The listing builds one solid part. Answer for the finished solid, in the listing's coordinates (mm). Round coordinates to 2 decimals unless told otherwise and drop trailing zeros. Write each loop counter-clockwise with the first axis right and the second up, starting at its lowest first coordinate (ties: lowest second). Pieces come first, ordered by that corner, then holes. Notation, with made-up numbers: (26, 67) - (70, 67) arc R6 ccw to (70, 76) - close; hole circle Ø3 at (-24, 52). An arc over 180 degrees is marked (long way). Answer as CSV lines item,"result". Start each with the question number.
Item 1: Flat-ended cylindrical pins translate along their axes: pin 1 (1 mm diameter, centred on x = -13.5, z = 39, fed in from -Y); pin 2 (2 mm diameter, centred on x = 33, y = 13.5, fed in from +Z); pin 3 (2 mm diameter, centred on x = 11.5, y = -21.5, fed in from -Z). Find the tip coordinate at first contact, or state that the pin passes through.
Item 2: A cutting plane is placed at A-A on y = 7. Determine the outline of the cut face in (x, z), and give its area (3 significant figures).
Item 3: Straight lines are drawn through the part: line 1 along Z through (x, y) = (28.5, 29); line 2 along Z through (x, y) = (30.5, -8); line 3 along Y through (x, z) = (-17, 26.5). For each, find the intervals that lie inside material, in ascending order. Write a range as [from, to].
Item 4: A cutting plane is placed at B-B on z = -24. Determine the outline of the cut face in (x, y).
Item 5: A cutting plane is placed at C-C on x = 32. Determine the outline of the cut face in (y, z).
Item 6: A cutting plane is placed at D-D on y = 31.5. Determine the outline of the cut face in (x, z), and give its area (3 significant figures).
```python
from build123d import *

# Parameters (mm, degrees)
F12_DEPTH      = 37.3243635206
F12_DEPTH_BACK = 37.3243635206
F15_DEPTH      = 37.3243635206
F15_DEPTH_BACK = 37.3243635206
F18_DEPTH      = 37.3243635206
F18_DEPTH_BACK = 37.3243635206
F21_DEPTH      = 37.3243635206
F21_DEPTH_BACK = 37.3243635206
F24_DEPTH      = 37.3243635206
F24_DEPTH_BACK = 37.3243635206
F28_DEPTH      = 99.1671965959
F28_DEPTH_BACK = 99.1671965959
F32_DEPTH      = 89.4601183415
F32_DEPTH_BACK = 89.4601183415
F35_DEPTH      = 89.4601183415
F35_DEPTH_BACK = 88.5596960493
F39_DEPTH      = 99.1671965959
F39_DEPTH_BACK = 96.8098604305
F42_DEPTH      = 68.0823305395
F42_DEPTH_BACK = 70.9961582856
F45_DEPTH      = 92.4043169267
F45_DEPTH_BACK = 99.1671965959
F48_DEPTH      = 81.4313769211
F48_DEPTH_BACK = 89.4601183415
F52_DEPTH      = 88.5596960493
F52_DEPTH_BACK = 82.3317992133
F56_DEPTH      = 92.4043169267
F56_DEPTH_BACK = 96.8098604305
F59_DEPTH      = 68.0823305395
F59_DEPTH_BACK = 68.0823305395
F62_DEPTH      = 37.3243635206
F62_DEPTH_BACK = 37.3243635206
F65_DEPTH      = 68.0823305395
F65_DEPTH_BACK = 68.0823305395
F68_DEPTH      = 81.4313769211
F68_DEPTH_BACK = 81.4313769211
F71_DEPTH      = 92.4043169267
F71_DEPTH_BACK = 92.4043169267
F74_DEPTH      = 92.4043169267
F74_DEPTH_BACK = 92.4043169267


# Not quite as in the source:
# - a feature names something its author has since deleted; it is built from what else it names


with BuildPart() as f9:
    # F7 (on Front) → F9 (revolve)
    with BuildSketch(Plane.XZ):
        with BuildLine():
            Line((0, 0), (0, 31.75))
            Line((0, 31.75), (0, 70.9951582856))
            ThreePointArc((0, 70.9951582856), (-70.9951582856, 0), (0, -70.9951582856))
            Line((0, -70.9951582856), (0, -31.75))
            Line((0, -31.75), (0, 0))
        make_face()
    revolve(axis=Axis((0, 0, -35.4975791428), (0, 0, -1)))

    # F11 (on 3pt) → F12 (cut, two sides)
    with BuildSketch(Plane(origin=(0, 0, 0), x_dir=(-0.5877852523, 0.8090169944, 0), z_dir=(0.8090169944, 0.5877852523, 0))) as f12_sk:
        Polygon((-63.5, -70.9951582856), (0, -70.9951582856), (-51.3725791428, -31.75), (-63.5, -31.75), align=None)
    extrude(amount=F12_DEPTH, mode=Mode.SUBTRACT)
    extrude(f12_sk.sketch, amount=-F12_DEPTH_BACK, mode=Mode.SUBTRACT)

    # F14 (on 3pt) → F15 (cut, two sides)
    with BuildSketch(Plane(origin=(0, 0, 0), x_dir=(-0.5877852523, -0.8090169944, 0), z_dir=(-0.8090169944, 0.5877852523, 0))) as f15_sk:
        Polygon((51.3725791428, -31.75), (0, -70.9951582856), (63.5, -70.9951582856), (63.5, -31.75), align=None)
    extrude(amount=-F15_DEPTH, mode=Mode.SUBTRACT)
    extrude(f15_sk.sketch, amount=F15_DEPTH_BACK, mode=Mode.SUBTRACT)

    # F17 (on 3pt) → F18 (cut, two sides)
    with BuildSketch(Plane(origin=(0, 0, 0), x_dir=(0.9510565163, -0.3090169944, 0), z_dir=(-0.3090169944, -0.9510565163, 0))) as f18_sk:
        Polygon((-63.5, -70.9951582856), (0, -70.9951582856), (-51.3725791428, -31.75), (-63.5, -31.75), align=None)
    extrude(amount=-F18_DEPTH, mode=Mode.SUBTRACT)
    extrude(f18_sk.sketch, amount=F18_DEPTH_BACK, mode=Mode.SUBTRACT)

    # F20 (on 3pt) → F21 (cut, two sides)
    with BuildSketch(Plane.YZ) as f21_sk:
        Polygon((51.3725791428, -31.75), (0, -70.9951582856), (63.5, -70.9951582856), (63.5, -31.75), align=None)
    extrude(amount=-F21_DEPTH, mode=Mode.SUBTRACT)
    extrude(f21_sk.sketch, amount=F21_DEPTH_BACK, mode=Mode.SUBTRACT)

    # F23 (on 3pt) → F24 (cut, two sides)
    with BuildSketch(Plane(origin=(0, 0, 0), x_dir=(-0.9510565163, -0.3090169944, 0), z_dir=(-0.3090169944, 0.9510565163, 0))) as f24_sk:
        Polygon((-63.5, -70.9951582856), (0, -70.9951582856), (-51.3725791428, -31.75), (-63.5, -31.75), align=None)
    extrude(amount=F24_DEPTH, mode=Mode.SUBTRACT)
    extrude(f24_sk.sketch, amount=-F24_DEPTH_BACK, mode=Mode.SUBTRACT)

    # F27 (on 3pt) → F28 (cut, two sides)
    with BuildSketch(Plane(origin=(0, 0, 0), x_dir=(-0.5877852523, 0.8090169944, 0), z_dir=(0.8090169944, 0.5877852523, 0))) as f28_sk:
        Polygon((-70.9951582856, -31.75), (-51.3725791428, -31.75), (-63.5, 31.75), (-70.9951582856, 31.75), align=None)
    extrude(amount=F28_DEPTH, mode=Mode.SUBTRACT)
    extrude(f28_sk.sketch, amount=-F28_DEPTH_BACK, mode=Mode.SUBTRACT)

    # F31 (on 3pt) → F32 (cut, two sides)
    with BuildSketch(Plane(origin=(0, 0, 0), x_dir=(0.9510565163, -0.3090169944, 0), z_dir=(-0.3090169944, -0.9510565163, 0))) as f32_sk:
        Polygon((70.9951582856, 31.75), (51.3725791428, 31.75), (63.5, -31.75), (70.9951582856, -31.75), align=None)
    extrude(amount=-F32_DEPTH, mode=Mode.SUBTRACT)
    extrude(f32_sk.sketch, amount=F32_DEPTH_BACK, mode=Mode.SUBTRACT)

    # F34 (on 3pt) → F35 (cut, two sides)
    with BuildSketch(Plane(origin=(0, 0, 0), x_dir=(0.9510565163, 0.3090169944, 0), z_dir=(0.3090169944, -0.9510565163, 0))) as f35_sk:
        Polygon((63.5, 31.75), (51.3725791428, -31.75), (70.9951582856, -31.75), (70.9951582856, 31.75), align=None)
    extrude(amount=-F35_DEPTH, mode=Mode.SUBTRACT)
    extrude(f35_sk.sketch, amount=F35_DEPTH_BACK, mode=Mode.SUBTRACT)

    # F38 (on 3pt) → F39 (cut, two sides)
    with BuildSketch(Plane(origin=(0, 0, 0), x_dir=(0.5877852523, 0.8090169944, 0), z_dir=(0.8090169944, -0.5877852523, 0))) as f39_sk:
        Polygon((70.9951582856, 31.75), (51.3725791428, 31.75), (63.5, -31.75), (70.9951582856, -31.75), align=None)
    extrude(amount=-F39_DEPTH, mode=Mode.SUBTRACT)
    extrude(f39_sk.sketch, amount=F39_DEPTH_BACK, mode=Mode.SUBTRACT)

    # F41 (on 3pt) → F42 (cut, two sides)
    with BuildSketch(Plane(origin=(0, 0, 0), x_dir=(0, -1, 0), z_dir=(-1, 0, 0))) as f42_sk:
        Polygon((-70.9951582856, -31.75), (-51.3725791428, -31.75), (-63.5, 31.75), (-70.9951582856, 31.75), align=None)
    extrude(amount=-F42_DEPTH, mode=Mode.SUBTRACT)
    extrude(f42_sk.sketch, amount=F42_DEPTH_BACK, mode=Mode.SUBTRACT)

    # F44 (on 3pt) → F45 (cut, two sides)
    with BuildSketch(Plane(origin=(0, 0, 0), x_dir=(0.5877852523, -0.8090169944, 0), z_dir=(-0.8090169944, -0.5877852523, 0))) as f45_sk:
        Polygon((-63.5, -31.75), (-51.3725791428, 31.75), (-70.9951582856, 31.75), (-70.9951582856, -31.75), align=None)
    extrude(amount=-F45_DEPTH, mode=Mode.SUBTRACT)
    extrude(f45_sk.sketch, amount=F45_DEPTH_BACK, mode=Mode.SUBTRACT)

    # F47 (on 3pt) → F48 (cut, two sides)
    with BuildSketch(Plane(origin=(0, 0, 0), x_dir=(0.9510565163, -0.3090169944, 0), z_dir=(-0.3090169944, -0.9510565163, 0))) as f48_sk:
        Polygon((-70.9951582856, -31.75), (-51.3725791428, -31.75), (-63.5, 31.75), (-70.9951582856, 31.75), align=None)
    extrude(amount=-F48_DEPTH, mode=Mode.SUBTRACT)
    extrude(f48_sk.sketch, amount=F48_DEPTH_BACK, mode=Mode.SUBTRACT)

    # F51 (on 3pt) → F52 (cut, two sides)
    with BuildSketch(Plane(origin=(0, 0, 0), x_dir=(-0.9510565163, -0.3090169944, 0), z_dir=(-0.3090169944, 0.9510565163, 0))) as f52_sk:
        Polygon((70.9951582856, 31.75), (51.3725791428, 31.75), (63.5, -31.75), (70.9951582856, -31.75), align=None)
    extrude(amount=-F52_DEPTH, mode=Mode.SUBTRACT)
    extrude(f52_sk.sketch, amount=F52_DEPTH_BACK, mode=Mode.SUBTRACT)

    # F55 (on 3pt) → F56 (cut, two sides)
    with BuildSketch(Plane(origin=(0, 0, 0), x_dir=(0.5877852523, 0.8090169944, 0), z_dir=(0.8090169944, -0.5877852523, 0))) as f56_sk:
        Polygon((-70.9951582856, -31.75), (-51.3725791428, -31.75), (-63.5, 31.75), (-70.9951582856, 31.75), align=None)
    extrude(amount=-F56_DEPTH, mode=Mode.SUBTRACT)
    extrude(f56_sk.sketch, amount=F56_DEPTH_BACK, mode=Mode.SUBTRACT)

    # F58 (on 3pt) → F59 (cut, two sides)
    with BuildSketch(Plane(origin=(0, 0, 0), x_dir=(0, -1, 0), z_dir=(-1, 0, 0))) as f59_sk:
        Polygon((70.9951582856, 31.75), (51.3725791428, 31.75), (63.5, -31.75), (70.9951582856, -31.75), align=None)
    extrude(amount=-F59_DEPTH, mode=Mode.SUBTRACT)
    extrude(f59_sk.sketch, amount=F59_DEPTH_BACK, mode=Mode.SUBTRACT)

    # F61 (on 3pt) → F62 (cut, two sides)
    with BuildSketch(Plane(origin=(0, 0, 0), x_dir=(0.9510565163, -0.3090169944, 0), z_dir=(-0.3090169944, -0.9510565163, 0))) as f62_sk:
        Polygon((63.5, 70.9951582856), (0, 70.9951582856), (51.3725791428, 31.75), (63.5, 31.75), align=None)
    extrude(amount=F62_DEPTH, mode=Mode.SUBTRACT)
    extrude(f62_sk.sketch, amount=-F62_DEPTH_BACK, mode=Mode.SUBTRACT)

    # F64 (on 3pt) → F65 (cut, two sides)
    with BuildSketch(Plane.YZ) as f65_sk:
        Polygon((-51.3725791428, 31.75), (0, 70.9951582856), (-63.5, 70.9951582856), (-63.5, 31.75), align=None)
    extrude(amount=-F65_DEPTH, mode=Mode.SUBTRACT)
    extrude(f65_sk.sketch, amount=F65_DEPTH_BACK, mode=Mode.SUBTRACT)

    # F67 (on 3pt) → F68 (cut, two sides)
    with BuildSketch(Plane(origin=(0, 0, 0), x_dir=(0.9510565163, 0.3090169944, 0), z_dir=(0.3090169944, -0.9510565163, 0))) as f68_sk:
        Polygon((-51.3725791428, 31.75), (0, 70.9951582856), (-63.5, 70.9951582856), (-63.5, 31.75), align=None)
    extrude(amount=-F68_DEPTH, mode=Mode.SUBTRACT)
    extrude(f68_sk.sketch, amount=F68_DEPTH_BACK, mode=Mode.SUBTRACT)

    # F70 (on 3pt) → F71 (cut, two sides)
    with BuildSketch(Plane(origin=(0, 0, 0), x_dir=(-0.5877852523, 0.8090169944, 0), z_dir=(0.8090169944, 0.5877852523, 0))) as f71_sk:
        Polygon((63.5, 70.9951582856), (0, 70.9951582856), (51.3725791428, 31.75), (63.5, 31.75), align=None)
    extrude(amount=-F71_DEPTH, mode=Mode.SUBTRACT)
    extrude(f71_sk.sketch, amount=F71_DEPTH_BACK, mode=Mode.SUBTRACT)

    # F73 (on 3pt) → F74 (cut, two sides)
    with BuildSketch(Plane(origin=(0, 0, 0), x_dir=(0.5877852523, 0.8090169944, 0), z_dir=(0.8090169944, -0.5877852523, 0))) as f74_sk:
        Polygon((63.5, 70.9951582856), (0, 70.9951582856), (51.3725791428, 31.75), (63.5, 31.75), align=None)
    extrude(amount=-F74_DEPTH, mode=Mode.SUBTRACT)
    extrude(f74_sk.sketch, amount=F74_DEPTH_BACK, mode=Mode.SUBTRACT)


solid = f9.part
```
Geometry says:
1,pin 1,"stops at y = -42.54"
1,pin 2,"stops at z = 48.6"
1,pin 3,"stops at z = -53.31"
2,outline,"(-60.39, 11.33) - (-51.74, -31.75) - (-5.09, -65.65) - (5.09, -65.65) - (51.74, -31.75) - (60.39, 11.33) - (56.29, 31.75) - (21.54, 57) - (0, 66.67) - (-21.54, 57) - (-56.29, 31.75) - close"
2,area,"11,300 mm^2"
3,line 1,"z = [-43.44, 40.27]"
3,line 2,"z = [-50.72, 46.95]"
3,line 3,"y = [-52.38, 52.39]"
4,outline,"(-60.39, -14.83) - (-57.58, -23.5) - (-4.56, -62.02) - (4.56, -62.02) - (57.58, -23.5) - (60.39, -14.83) - (40.14, 47.5) - (32.77, 52.85) - (-32.77, 52.85) - (-40.14, 47.5) - close"
5,outline,"(-53.1, 22.69) - (-40.25, -31.75) - (-10.4, -50.2) - (44.04, -37.35) - (51.37, -31.75) - (53.1, -22.69) - (40.25, 31.75) - (10.4, 50.2) - (-44.04, 37.35) - (-51.37, 31.75) - close"
6,outline,"(-51.76, 8) - (-43.78, -31.75) - (-22.89, -46.93) - (22.89, -46.93) - (43.78, -31.75) - (51.76, 8) - (44.04, 31.75) - (0, 51.53) - (-44.04, 31.75) - close"
6,area,"7,960 mm^2"
